```python
from build123d import *

# Parameters (mm, degrees)
F0_R     = 4.25
F1_DEPTH = 5.5
F3_DEPTH = 3
F4_R     = 2.5
F5_DEPTH = 25


with BuildPart() as f1:
    # F0 (on Front) → F1 (new body)
    with BuildSketch(Plane.XZ):
        Circle(F0_R)
    extrude(amount=F1_DEPTH)

    # F2 (on face) → F3 (cut)
    with BuildSketch(Plane.XZ.offset(5.5)):
        Polygon((3.151009, 1.714376), (0, 3.066219), (0, 0), (3.151009, 0), align=None)
        Polygon((0, 0), (0, 3.066219), (-3.151009, 1.714376), (-3.151009, 0), align=None)
        Polygon((3.151009, 0), (0, 0), (0, -3.066219), (3.151009, -1.714376), align=None)
        Polygon((0, -3.066219), (0, 0), (-3.151009, 0), (-3.151009, -1.714376), align=None)
    extrude(amount=-F3_DEPTH, mode=Mode.SUBTRACT)

    # F4 (on face) → F5 (join)
    with BuildSketch(Plane(origin=(0, 0, 0), x_dir=(-1, 0, 0), z_dir=(0, 1, 0))):
        Circle(F4_R)
    extrude(amount=F5_DEPTH)


solid = f1.part
```
Geometry check sheet. Reference: the model listing, model coordinates, mm. A direction names the side the tool comes from. Coordinates: 2 decimals unless noted, no trailing zeros. Order: outer loops, then holes, each group sorted by start corner. A loop starts at its lowest first (then second) coordinate and runs counter-clockwise, first axis right, second up. Notation, with made-up numbers: (21.5, 42.5) - (39.5, 42.5) arc R11 cw to (39.5, 52.5) - close; hole circle Ø11 at (-39, -13). An arc over 180 degrees is marked (long way). Answer in a Markdown table with one row per item. Add a question column.
1. Draft check along X on faces 1 (the face through (0, -2.5, 0)), 2 (the face through (0.54, 12.32, -2.44)), 3 (the face through (1, -5.5, -3)). Enter one of: +X half, -X half, draft (parallel to the pull), parting line (faces both ways), or undercut.
2. Section check B-B (z = 0). Enter the section's corners in (x, y), plus the area to 3 significant figures.
3. Section check A-A (y = -3). Enter the section's corners in (x, z).
4. Gauge pin test, flat ends, axial feed: pin 1 Ø2 at (y, z) = (1.5, 2) entering from -X; pin 2 Ø1 at (x, y) = (-3, -2.5) entering from -Z; pin 3 Ø4 at (y, z) = (5.5, 0.5) entering from +X. Record the tip position at first contact, or that the pin passes through.
5. Material ranges on L1, parallel to Y at x = 0.75, z = 0.25; L2, parallel to Y at x = -2.75, z = 2.25; L3, parallel to Z at x = -0.5, y = -4, recorded low to high. Write a range as [from, to].
6. Section check C-C (y = 18). Enter the section's corners in (x, z).
7. Section check D-D (x = -3.5). Enter the section's corners in (y, z), plus the area to 3 significant figures.
8. Access from +Z, -Z, +X, -X, +Y, -Y to the whole of each face (thin tool, end or side, straight path). Record for faces 4 (the face through (2, 0, -2)), 5 (the face through (1.55, -4.02, -2.4)), 6 (the face through (2.285, -2.712, 3.584)).
Data:
| question | item | result |
|---|---|---|
| 1 | face 1 | undercut |
| 1 | face 2 | parting line |
| 1 | face 3 | draft |
| 2 | outline | (-4.25, -5.5) - (-3.15, -5.5) - (-3.15, -2.5) - (3.15, -2.5) - (3.15, -5.5) - (4.25, -5.5) - (4.25, 0) - (2.5, 0) - (2.5, 25) - (-2.5, 25) - (-2.5, 0) - (-4.25, 0) - close |
| 2 | area | 153 mm² |
| 3 | outline | circle Ø8.5 at (0, 0); hole (-3.15, -1.71) - (0, -3.07) - (3.15, -1.71) - (3.15, 1.71) - (0, 3.07) - (-3.15, 1.71) - close |
| 4 | pin 1 | stops at x = -2.29 |
| 4 | pin 2 | stops at z = -3.44 |
| 4 | pin 3 | stops at x = 2.5 |
| 5 | L1 | y = [-2.5, 25] |
| 5 | L2 | y = [-5.5, 0] |
| 5 | L3 | z = [-4.22, -2.85], [2.85, 4.22] |
| 6 | outline | circle Ø5 at (0, 0) |
| 7 | outline | (-5.5, -2.41) - (0, -2.41) - (0, 2.41) - (-5.5, 2.41) - close |
| 7 | area | 26.5 mm² |
| 8 | face 4 | +Y |
| 8 | face 5 | -Y |
| 8 | face 6 | +Y, -Y |
